For this review, use the dimensioned drawing (mm, ordinates from the lowest corner) and the shaded views. Give positions to 0.01 mm unless a question says otherwise; leave off trailing zeros. Order: outer loops, then holes, each group sorted by start corner. A loop starts at its lowest first (then second) coordinate and runs counter-clockwise, first axis right, second up. Notation, with made-up numbers: (82, 4) - (132, 4) arc R18 cw to (132, 37) - close; hole circle Ø3 at (73.5, -34.75). An arc over 180 degrees is marked (long way). Use a Markdown table: item, result. Add a question column.
1) We need section C-C on x = 2.25. Write out the cut boundary in (y, z), then the cut area to 3 significant figures.
2) Wall thickness on L1, parallel to Y at x = 21.5, z = 2.3; L2, parallel to Y at x = 15, z = 2.05; L3, parallel to X at y = 2.5, z = 2.7: over which ranges is each line inside the solid? List them lowest first.
3) We need section B-B on z = 0.85. Give the number of separate pieces and of enclosed holes in the cut face, then the cut area to 3 significant figures.
4) Clearance check with flat-ended pins moving along their axes: P1, Ø1.5, axis at x = 13.5, z = 2, coming from the +Y side; P2, Ø0.9, axis at x = 21.5, y = 17.25, coming from the +Z side; P3, Ø0.9, axis at x = 2.5, z = 1.5, coming from the -Y side; P4, Ø1.7, axis at x = 15, y = 28.5, coming from the +Z side. State where each tip first meets the part, or that it passes through.
5) We need section A-A on y = 24.75. Write out the cut boundary in (x, z) (1 decimal).
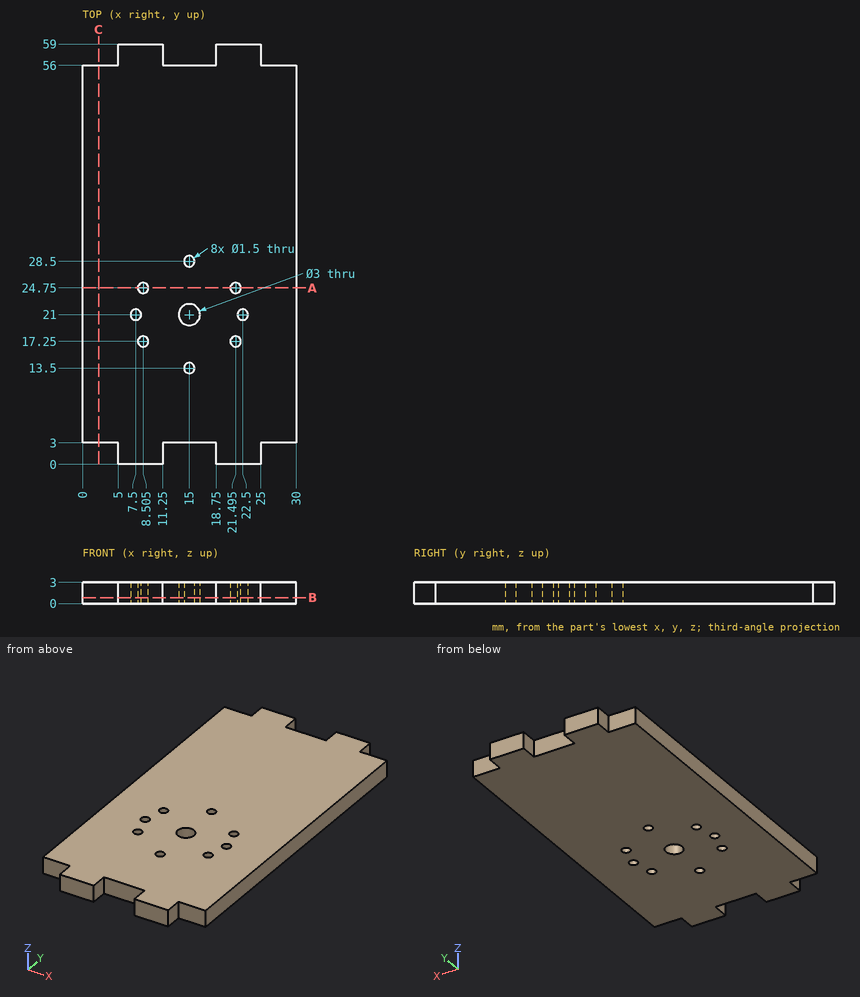
Checked values:
| question | item | result |
|---|---|---|
| 1 | outline | (3, 0) - (56, 0) - (56, 3) - (3, 3) - close |
| 1 | area | 159 mm² |
| 2 | L1 | 0 to 16.5, 18 to 24, 25.5 to 59 |
| 2 | L2 | 3 to 12.75, 14.25 to 19.5, 22.5 to 27.75, 29.25 to 56 |
| 2 | L3 | 5 to 11.25, 18.75 to 25 |
| 3 | separate pieces | 1 |
| 3 | enclosed holes | 9 |
| 3 | area | 1,640 mm² |
| 4 | P1 | y = 56 |
| 4 | P2 | through |
| 4 | P3 | y = 3 |
| 4 | P4 | z = 3 |
| 5 | outline | (0, 0) - (7.8, 0) - (7.8, 3) - (0, 3) - close; (9.3, 0) - (20.7, 0) - (20.7, 3) - (9.3, 3) - close; (22.2, 0) - (30, 0) - (30, 3) - (22.2, 3) - close |
